The model under review builds one solid part; all positions refer to its coordinate system, in mm. A direction names the side the tool comes from. Coordinates: 2 decimals unless noted, no trailing zeros. Loops run counter-clockwise (first coordinate to the right, second up) from the corner with the lowest first, then second, coordinate; pieces in that order, holes last. Notation, with made-up numbers: M 46.5,-13 L 86.5,-13 A19 ccw 86.5,-4 Z; hole C 32.25,69 d3. An arc over 180 degrees is marked long. Use CSV: the item, a comma, the result in double quotes. Start each with the question number.
from build123d import *

# Parameters (mm, degrees)
BOSS_EXTRUDE1_DEPTH  = 100
BOSS_EXTRUDE2_DEPTH  = 8
BOSS_EXTRUDE3_DEPTH  = 8
SKETCH10_R           = 2
CUT_EXTRUDE4_DEPTH   = 8.75
SKETCH11_W           = 7.8
SKETCH11_H           = 2.8
CUT_EXTRUDE5_DEPTH   = 101.180739791
CUT_EXTRUDE1_REACH   = 111.927
SKETCH5_R            = 3
SKETCH6_W            = 14
SKETCH6_H            = 10
CUT_EXTRUDE2_DEPTH   = 6
BOSS_EXTRUDE4_DEPTH  = 10
BOSS_EXTRUDE11_DEPTH = 10
CUT_EXTRUDE3_REACH   = 131.325
SKETCH9_R            = 1.5


with BuildPart() as part:
    # Sketch1 → Boss-Extrude1 (new body)
    with BuildSketch(Plane(origin=(0, 0, 0), x_dir=(0, 0, -1), z_dir=(1, 0, 0))):
        Polygon((0, 0), (40, 0), (40, 12), (38.5, 12), (38.5, 6), (25, 6), (25, 12), (23.5, 12), (23.5, 6), (16.5, 6), (16.5, 12), (15, 12), (15, 6), (1.5, 6), (1.5, 12), (0, 12), align=None)
    extrude(amount=BOSS_EXTRUDE1_DEPTH)

    # Sketch2 → Boss-Extrude2 (add)
    with BuildSketch(Plane(origin=(18.825, 0, 0), x_dir=(0, 0, -1), z_dir=(1, 0, 0))):
        Polygon((15, 6), (15, 12), (8, 13.5), (8, 22), (32, 22), (32, 13.5), (25, 12), (25, 6), align=None)
    extrude(amount=-BOSS_EXTRUDE2_DEPTH)

    # Sketch4 → Boss-Extrude3 (add)
    with BuildSketch(Plane(origin=(59.625, 0, 0), x_dir=(0, 0, -1), z_dir=(1, 0, 0))):
        Polygon((25, 6), (15, 6), (15, 12), (8, 13.5), (8, 22), (32, 22), (32, 13.5), (25, 12), align=None)
    extrude(amount=BOSS_EXTRUDE3_DEPTH)

    # Sketch10 → Cut-Extrude4 (cut)
    with BuildSketch(Plane(origin=(0, 22, 0), x_dir=(1, 0, 0), z_dir=(0, 1, 0))):
        with Locations(Location((14.475, 14.625, 0), (0, 0, 270))):
            Circle(SKETCH10_R)
        with Locations(Location((14.475, 25.375, 0), (0, 0, 270))):
            Circle(SKETCH10_R)
        with Locations(Location((63.975, 14.625, 0), (0, 0, 270))):
            Circle(SKETCH10_R)
        with Locations(Location((63.975, 25.375, 0), (0, 0, 270))):
            Circle(SKETCH10_R)
    extrude(amount=-CUT_EXTRUDE4_DEPTH, mode=Mode.SUBTRACT)

    # Sketch11 → Cut-Extrude5 (cut, through all)
    with BuildSketch(Plane.ZY.offset(-10.825)):
        with Locations((-25.375, 17.6)):
            Rectangle(SKETCH11_W, SKETCH11_H)
        with Locations((-14.625, 17.6)):
            Rectangle(SKETCH11_W, SKETCH11_H)
    extrude(amount=-CUT_EXTRUDE5_DEPTH, mode=Mode.SUBTRACT)

    # Sketch5 → Cut-Extrude1 (cut, up to next)
    with BuildSketch(Plane.XZ, mode=Mode.PRIVATE) as cut_extrude1_sk1:
        with Locations(Location((50, -20, 0), (0, 0, 270))):
            Circle(SKETCH5_R)
    cut_extrude1_tool1 = extrude(cut_extrude1_sk1.sketch, amount=-CUT_EXTRUDE1_REACH, mode=Mode.PRIVATE) & part.part
    # Sketch5 → Cut-Extrude1 (cut, up to next)
    with BuildSketch(Plane.XZ, mode=Mode.PRIVATE) as cut_extrude1_sk2:
        with BuildLine():
            Line((8, -31), (92, -31))
            ThreePointArc((92, -31), (94.5, -33.5), (92, -36))
            Line((92, -36), (8, -36))
            ThreePointArc((8, -36), (5.5, -33.5), (8, -31))
        make_face()
    cut_extrude1_tool2 = extrude(cut_extrude1_sk2.sketch, amount=-CUT_EXTRUDE1_REACH, mode=Mode.PRIVATE) & part.part
    # Sketch5 → Cut-Extrude1 (cut, up to next)
    with BuildSketch(Plane.XZ, mode=Mode.PRIVATE) as cut_extrude1_sk3:
        with BuildLine():
            Line((92, -4), (8, -4))
            ThreePointArc((8, -4), (5.5, -6.5), (8, -9))
            Line((8, -9), (92, -9))
            ThreePointArc((92, -9), (94.5, -6.5), (92, -4))
        make_face()
    cut_extrude1_tool3 = extrude(cut_extrude1_sk3.sketch, amount=-CUT_EXTRUDE1_REACH, mode=Mode.PRIVATE) & part.part
    add(cut_extrude1_tool1.solids().sort_by_distance((50, 0, -20))[0], mode=Mode.SUBTRACT)
    add(cut_extrude1_tool2.solids().sort_by_distance((50, 0, -33.5))[0], mode=Mode.SUBTRACT)
    add(cut_extrude1_tool3.solids().sort_by_distance((50, 0, -6.5))[0], mode=Mode.SUBTRACT)

    # Sketch6 → Cut-Extrude2 (cut)
    with BuildSketch(Plane(origin=(0, 6, 0), x_dir=(1, 0, 0), z_dir=(0, 1, 0))):
        with Locations((50, 20)):
            Rectangle(SKETCH6_W, SKETCH6_H)
    extrude(amount=CUT_EXTRUDE2_DEPTH, mode=Mode.SUBTRACT)

    # Sketch7 → Boss-Extrude4 (add)
    with BuildSketch(Plane(origin=(100, 0, 0), x_dir=(0, 0, -1), z_dir=(1, 0, 0))):
        Polygon((0, 0), (40, 0), (40, 12), (40, 55), (10, 55), (0, 12), align=None)
        Polygon((35, 50), (13.970637222, 50), (5.13342792, 12), (35, 12), align=None, mode=Mode.SUBTRACT)
    extrude(amount=BOSS_EXTRUDE4_DEPTH)

    # Sketch8 → Boss-Extrude11 (add)
    with BuildSketch(Plane.ZY):
        Polygon((-40, 0), (-40, 55), (-10, 55), (0, 12), (0, 0), align=None)
        Polygon((-35, 50), (-13.970637222, 50), (-5.13342792, 12), (-35, 12), align=None, mode=Mode.SUBTRACT)
    extrude(amount=BOSS_EXTRUDE11_DEPTH)

    # Sketch9 → Cut-Extrude3 (cut, up to next)
    with BuildSketch(Plane(origin=(0, 0, -40), x_dir=(-1, 0, 0), z_dir=(0, 0, -1)), mode=Mode.PRIVATE) as cut_extrude3_sk1:
        with Locations((-105, 45)):
            Circle(SKETCH9_R)
    cut_extrude3_tool1 = extrude(cut_extrude3_sk1.sketch, amount=-CUT_EXTRUDE3_REACH, mode=Mode.PRIVATE) & part.part
    # Sketch9 → Cut-Extrude3 (cut, up to next)
    with BuildSketch(Plane(origin=(0, 0, -40), x_dir=(-1, 0, 0), z_dir=(0, 0, -1)), mode=Mode.PRIVATE) as cut_extrude3_sk2:
        with Locations((-105, 32.5)):
            Circle(SKETCH9_R)
    cut_extrude3_tool2 = extrude(cut_extrude3_sk2.sketch, amount=-CUT_EXTRUDE3_REACH, mode=Mode.PRIVATE) & part.part
    # Sketch9 → Cut-Extrude3 (cut, up to next)
    with BuildSketch(Plane(origin=(0, 0, -40), x_dir=(-1, 0, 0), z_dir=(0, 0, -1)), mode=Mode.PRIVATE) as cut_extrude3_sk3:
        with Locations((-105, 17.5)):
            Circle(SKETCH9_R)
    cut_extrude3_tool3 = extrude(cut_extrude3_sk3.sketch, amount=-CUT_EXTRUDE3_REACH, mode=Mode.PRIVATE) & part.part
    # Sketch9 → Cut-Extrude3 (cut, up to next)
    with BuildSketch(Plane(origin=(0, 0, -40), x_dir=(-1, 0, 0), z_dir=(0, 0, -1)), mode=Mode.PRIVATE) as cut_extrude3_sk4:
        with Locations((5, 45)):
            Circle(SKETCH9_R)
    cut_extrude3_tool4 = extrude(cut_extrude3_sk4.sketch, amount=-CUT_EXTRUDE3_REACH, mode=Mode.PRIVATE) & part.part
    # Sketch9 → Cut-Extrude3 (cut, up to next)
    with BuildSketch(Plane(origin=(0, 0, -40), x_dir=(-1, 0, 0), z_dir=(0, 0, -1)), mode=Mode.PRIVATE) as cut_extrude3_sk5:
        with Locations((5, 32.5)):
            Circle(SKETCH9_R)
    cut_extrude3_tool5 = extrude(cut_extrude3_sk5.sketch, amount=-CUT_EXTRUDE3_REACH, mode=Mode.PRIVATE) & part.part
    # Sketch9 → Cut-Extrude3 (cut, up to next)
    with BuildSketch(Plane(origin=(0, 0, -40), x_dir=(-1, 0, 0), z_dir=(0, 0, -1)), mode=Mode.PRIVATE) as cut_extrude3_sk6:
        with Locations((5, 17.5)):
            Circle(SKETCH9_R)
    cut_extrude3_tool6 = extrude(cut_extrude3_sk6.sketch, amount=-CUT_EXTRUDE3_REACH, mode=Mode.PRIVATE) & part.part
    add(cut_extrude3_tool1.solids().sort_by_distance((105, 45, -40))[0], mode=Mode.SUBTRACT)
    add(cut_extrude3_tool2.solids().sort_by_distance((105, 32.5, -40))[0], mode=Mode.SUBTRACT)
    add(cut_extrude3_tool3.solids().sort_by_distance((105, 17.5, -40))[0], mode=Mode.SUBTRACT)
    add(cut_extrude3_tool4.solids().sort_by_distance((-5, 45, -40))[0], mode=Mode.SUBTRACT)
    add(cut_extrude3_tool5.solids().sort_by_distance((-5, 32.5, -40))[0], mode=Mode.SUBTRACT)
    add(cut_extrude3_tool6.solids().sort_by_distance((-5, 17.5, -40))[0], mode=Mode.SUBTRACT)


solid = part.part
1. Add section C-C (y = 7.5). Give the number of separate pieces and of enclosed holes in the cut face, plus the area to 3 significant figures.
2. Add section B-B (x = 105). Write out the cut boundary in (y, z).
3. Insertion check: pin 1 Ø6.5 at (x, z) = (63.975, -14.625) entering from +Y; pin 2 Ø1.4 at (x, y) = (62.5, 18.5) entering from +Z; pin 3 Ø8 at (x, z) = (94, -4.5) entering from +Y. Each pin has a flat end and moves straight along its axis. Give the tip position at first contact, or say it passes through.
4. To check wall thickness, follow line 1 along Y through (x, z) = (-5, -37.1); line 2 along X through (y, z) = (11, -32); line 3 along X through (y, z) = (44, -38). State the ranges of each line that lie inside material, in increasing order.
5. Draft analysis for pull direction Y (two halves, no side actions). For faces 1 (the flat face through (-4.93, 33.8, -5.07)), 2 (the cylindrical face through (5.5, 3, -33.6)), 3 (the flat face through (-4.93, 31.266, -9.614)), state which applies: released by +Y, released by -Y, zero draft, split by the parting line, or undercut.
6. Add section D-D (x = 50). Write out the cut boundary in (y, z), plus the area to 3 significant figures.
7. Add section A-A (z = -20). Write out the cut boundary in (x, y) (3 decimals).
8. For faces 4 (the flat face through (31, 9, -23.5)), 5 (the flat face through (105, 55, -25)), 6 (the flat face through (17, 16.2, -15)), 7 (the flat face through (51, 3, -4)), 8 (the flat face through (-4, 12, -20)), list the 3-axis set-ups (+Z, -Z, +X, -X, +Y, -Y) from which the entire face can be reached by the end or side of a thin tool; tool diameter is ignored.
Solved:
1,separate pieces,"1"
1,enclosed holes,"3"
1,area,"1,470 mm^2"
2,outline,"M 0,-40 L 16,-40 L 16,-35 L 12,-35 L 12,-5.13 L 50,-13.97 L 50,-35 L 46.5,-35 L 46.5,-40 L 55,-40 L 55,-10 L 12,0 L 0,0 Z; M 19,-40 L 31,-40 L 31,-35 L 19,-35 Z; M 34,-40 L 43.5,-40 L 43.5,-35 L 34,-35 Z"
3,pin 1,"stops at y = 22"
3,pin 2,"stops at z = -8"
3,pin 3,"stops at y = 12"
4,line 1,"y = 0 to 16, 19 to 31, 34 to 43.5, 46.5 to 55"
4,line 2,"x = -10 to 0, 100 to 110"
4,line 3,"x = -10 to -6.12, -3.88 to 0, 100 to 103.88, 106.12 to 110"
5,face 1,"released by +Y"
5,face 2,"zero draft"
5,face 3,"undercut"
6,outline,"M 0,-40 L 12,-40 L 12,-38.5 L 6,-38.5 L 6,-36 L 0,-36 Z; M 0,-31 L 6,-31 L 6,-23 L 0,-23 Z; M 0,-17 L 6,-17 L 6,-9 L 0,-9 Z; M 0,-4 L 6,-4 L 6,-1.5 L 12,-1.5 L 12,0 L 0,0 Z"
6,area,"162 mm^2"
7,outline,"M -10,0 L 47,0 L 47,6 L 18.825,6 L 18.825,22 L 10.825,22 L 10.825,6 L 0,6 L 0,12 L -10,12 Z; M -10,50 L 0,50 L 0,55 L -10,55 Z; M 53,0 L 110,0 L 110,12 L 100,12 L 100,6 L 67.625,6 L 67.625,22 L 59.625,22 L 59.625,6 L 53,6 Z; M 100,50 L 110,50 L 110,55 L 100,55 Z"
8,face 4,"+Y"
8,face 5,"+Z, -Z, +X, -X, +Y"
8,face 6,"+X, -X"
8,face 7,"+Y, -Y"
8,face 8,"-X"
